Verification items for the finished model (mm, model axes). A direction names the side the tool comes from. Round coordinates to 2 decimals unless told otherwise and drop trailing zeros. Order: outer loops, then holes, each group sorted by start corner. A loop starts at its lowest first (then second) coordinate and runs counter-clockwise, first axis right, second up. Notation, with made-up numbers: M -12.5,86.5 L 27.5,86.5 A8 cw 27.5,94.5 Z; hole C 47,81.5 d10. An arc over 180 degrees is marked long. Use one line per item in the form item = value. Start each with the question number.
Item 1: Release check for a two-part mould opening along Y. For faces 3 (the cylindrical face through (52.62, -4.69, 1.57)), 4 (the flat face through (37.17, 17, 1.57)), 5 (the cylindrical face through (57.105, 32.363, 1.565)) record: +Y half, -Y half, draft (parallel to the pull), parting line (faces both ways), or undercut.
Item 2: Cross-section at B-B on x = 45.72. Count the separate pieces of the cut face and the enclosed holes in it, then the cut area to 3 significant figures.
Item 3: Go/stop test with a flat-tipped pin: pin 1 Ø14.5 at (x, y) = (0, 0) entering from -Z. Record where the tip stops, or that it passes through.
Item 4: Tool access check on faces 1 (the flat face through (36.281, -16.002, 1.565)), 2 (the cylindrical face through (34.21, 21.42, 1.61)). Record the directions out of +Z, -Z, +X, -X, +Y, -Y that give a thin tool (end or side, any length) a straight path to the whole face; none if there is none.
Item 5: Thickness scan on probe 1 along X at (y, z) = (7, 1.7); probe 2 along Y at (x, z) = (19, 0.95); probe 3 along Y at (x, z) = (45.72, 0.95). Record the ranges inside material, lowest first. Write a range as [from, to].
Item 6: Cross-section at D-D on y = 54. Enter the section's corners in (x, z) (3 decimals).
Item 7: Cross-section at A-A on y = 0. Enter the section's corners in (x, z) (1 decimal).
from build123d import *

# Parameters (mm, degrees)
SKETCH2_R           = 7.9375
SKETCH2_R_2         = 3.2639
SKETCH2_R_3         = 4.191
BOSS_EXTRUDE1_DEPTH = 3.175
FILLET3_R           = 1.905
FILLET4_R           = 6.35
BOSS_EXTRUDE2_START = -3.175
BOSS_EXTRUDE2_DEPTH = 3.175
CUT_EXTRUDE1_DEPTH  = 12.065
FILLET5_R           = 3.175
CUT_EXTRUDE2_DEPTH  = 93.540316773


with BuildPart() as part:
    # Sketch2 → Boss-Extrude1 (new body)
    with BuildSketch(Plane.XY):
        with BuildLine():
            Line((22.709173353, -24.74146542), (50.237344688, -7.01528789))
            ThreePointArc((50.237344688, -7.01528789), (52.649254226, -4.648236557), (53.924522204, -1.51871084))
            ThreePointArc((53.924522204, -1.51871084), (57.106411985, 32.846575037), (54.035830718, 67.22198524))
            ThreePointArc((54.035830718, 67.22198524), (46.044632155, 72.608660166), (40.859194914, 64.485436554))
            Line((40.859194914, 64.485436554), (40.833827284, 64.453346951))
            ThreePointArc((40.833827284, 64.453346951), (30.975387354, 29.729811242), (-0.998479041, 12.979150429))
            ThreePointArc((-0.998479041, 12.979150429), (-12.595568055, 3.287395871), (-7.214067166, -10.835706769))
            Line((-7.214067166, -10.835706769), (13.567787564, -24.671601284))
            ThreePointArc((13.567787564, -24.671601284), (18.128061271, -26.069833859), (22.709173353, -24.74146542))
        make_face()
        Circle(SKETCH2_R, mode=Mode.SUBTRACT)
        with Locations((18.191828664, -17.726177531)):
            Circle(SKETCH2_R_2, mode=Mode.SUBTRACT)
        with Locations((45.72, 0)):
            Circle(SKETCH2_R_2, mode=Mode.SUBTRACT)
        with BuildLine():
            Line((40.584986991, 6.617553577), (21.318666843, -5.788581474))
            Line((21.318666843, -5.788581474), (11.074870198, -6.841239387))
            ThreePointArc((11.074870198, -6.841239387), (12.976194182, 1.036190528), (9.848859751, 8.512066016))
            ThreePointArc((9.848859751, 8.512066016), (23.445327069, 14.632175726), (34.749899024, 24.354640398))
            Line((34.749899024, 24.354640398), (40.584986991, 6.617553577))
        make_face(mode=Mode.SUBTRACT)
        with BuildLine():
            ThreePointArc((47.523781163, 56.501393309), (48.257752726, 32.370804269), (45.933946154, 8.34115665))
            Line((45.933946154, 8.34115665), (38.882442516, 29.775817606))
            ThreePointArc((38.882442516, 29.775817606), (45.039190515, 42.544935267), (47.523781163, 56.501393309))
        make_face(mode=Mode.SUBTRACT)
        with Locations((47.413333333, 66.018287029)):
            Circle(SKETCH2_R_3, mode=Mode.SUBTRACT)
    extrude(amount=BOSS_EXTRUDE1_DEPTH)

    # Fillet3
    fillet3_edges = [part.edges().sort_by_distance(p)[0] for p in [
        (45.933946154, 8.34115665, 1.5875),
        (47.523781163, 56.501393309, 1.5875),
    ]]
    fillet(fillet3_edges, radius=FILLET3_R)

    # Fillet4
    fillet4_edges = [part.edges().sort_by_distance(p)[0] for p in [
        (38.882442516, 29.775817606, 1.5875),
    ]]
    fillet(fillet4_edges, radius=FILLET4_R)

    # Sketch3 → Boss-Extrude2 (add)
    with BuildSketch(Plane.XY.offset(3.175).offset(BOSS_EXTRUDE2_START)):
        with BuildLine():
            ThreePointArc((37.967247274, 14.574773228), (38.850624387, 9.974362656), (38.539279751, 5.300264126))
            Line((38.539279751, 5.300264126), (40.584986991, 6.617553577))
            Line((40.584986991, 6.617553577), (37.967247274, 14.574773228))
        make_face()
        with BuildLine():
            ThreePointArc((14.005375904, -6.540099084), (13.004272705, -4.28056917), (12.890798124, -1.811802966))
            ThreePointArc((12.890798124, -1.811802966), (12.243860592, -4.42076736), (11.074870198, -6.841239387))
            Line((11.074870198, -6.841239387), (14.005375904, -6.540099084))
        make_face()
        with BuildLine():
            ThreePointArc((9.848859751, 8.512066016), (12.486736073, 3.679229335), (12.890798124, -1.811802966))
            ThreePointArc((12.890798124, -1.811802966), (16.379474961, 7.582660649), (23.480082515, 14.654307207))
            ThreePointArc((23.480082515, 14.654307207), (16.886076234, 11.091387544), (9.848859751, 8.512066016))
        make_face()
    extrude(amount=BOSS_EXTRUDE2_DEPTH)

    # Sketch4 → Cut-Extrude1 (cut)
    with BuildSketch(Plane.XY):
        with BuildLine():
            Line((38.539279751, 5.300264126), (24.727997063, 1.47053375))
            ThreePointArc((24.727997063, 1.47053375), (25.836206507, -0.508508416), (26.220294441, -2.743953008))
            ThreePointArc((26.220294441, -2.743953008), (24.044282761, -7.68479904), (18.930249644, -9.41501626))
            ThreePointArc((18.930249644, -9.41501626), (30.477911362, -6.56779892), (37.848176473, 2.766778194))
            ThreePointArc((37.848176473, 2.766778194), (38.239149826, 4.021130685), (38.539279751, 5.300264126))
        make_face()
        with BuildLine():
            ThreePointArc((24.727997063, 1.47053375), (17.733373474, 3.709866579), (12.890798123, -1.811802972))
            Line((12.890798123, -1.811802972), (24.727997063, 1.47053375))
        make_face()
        with BuildLine():
            Line((24.727997063, 1.47053375), (12.890798123, -1.811802972))
            ThreePointArc((12.890798123, -1.811802972), (14.27873169, -6.909589201), (18.930249644, -9.41501626))
            ThreePointArc((18.930249644, -9.41501626), (24.044282761, -7.68479904), (26.220294441, -2.743953008))
            ThreePointArc((26.220294441, -2.743953008), (25.836206507, -0.508508416), (24.727997063, 1.47053375))
        make_face()
    extrude(amount=CUT_EXTRUDE1_DEPTH, mode=Mode.SUBTRACT)

    # Fillet5
    fillet5_edges = [part.edges().sort_by_distance(p)[0] for p in [
        (34.749899024, 24.354640398, 1.5875),
    ]]
    fillet(fillet5_edges, radius=FILLET5_R)

    # Sketch5 → Cut-Extrude2 (cut, through all)
    with BuildSketch(Plane.XY.offset(3.175)):
        with BuildLine():
            Line((-7.214067166, -10.835706769), (-15.113040322, -22.700159224))
            Line((-15.113040322, -22.700159224), (13.567787564, -34.649979512))
            Line((13.567787564, -34.649979512), (13.567787564, -24.671601284))
            ThreePointArc((13.567787564, -24.671601284), (11.621320872, -22.869045851), (10.339065437, -20.546598936))
            ThreePointArc((10.339065437, -20.546598936), (6.247008791, -15.136046815), (-0.196937719, -13.01601021))
            ThreePointArc((-0.196937719, -13.01601021), (-3.862535324, -12.431256056), (-7.214067166, -10.835706769))
        make_face()
    extrude(amount=-CUT_EXTRUDE2_DEPTH, mode=Mode.SUBTRACT)


solid = part.part
Output values:
q1.face_3 = -Y half
q1.face_4 = undercut
q1.face_5 = parting line
q2.separate_pieces = 4
q2.enclosed_holes = 0
q2.area = 129 mm2
q3.pin_1 = through
q4.face_1 = +Z, -Z, +X, -Y
q4.face_2 = +Z, -Z
q5.probe_1 = [-10.98, -3.74], [3.74, 16.02], [38.79, 55.3]
q5.probe_2 = [-26.03, -20.89], [-14.56, -9.42], [10.94, 19.35]
q5.probe_3 = [-9.92, -3.26], [3.26, 14.91], [42.51, 62.18], [69.85, 72.53]
q6.outline = M 40.986,0 L 55.963,0 L 55.963,3.175 L 40.986,3.175 Z
q7.outline = M -13,0 L -7.9,0 L -7.9,3.2 L -13,3.2 Z; M 7.9,0 L 13.2,0 L 13.2,3.2 L 7.9,3.2 Z; M 36.6,0 L 42.5,0 L 42.5,3.2 L 36.6,3.2 Z; M 49,0 L 54.2,0 L 54.2,3.2 L 49,3.2 Z
